```python
from build123d import *

# Parameters (mm, degrees)
F1_DEPTH = 2


# Not quite as in the source:
# - a feature names something its author has since deleted; it is built from what else it names


with BuildPart() as f1:
    # F0 (on Top) → F1 (new body)
    with BuildSketch(Plane.XY):
        Polygon((27.5, 51.9615242271), (-27.5, 51.9615242271), (-27.5, 47.6313972081), (-25.5, 46.4766966698), (-25.5, 49.9615242271), (25.5, 49.9615242271), (25.5, 46.4766966698), (27.5, 47.6313972081), align=None)
        Polygon((-25.5, 46.4766966698), (-27.5, 47.6313972081), (-27.5, 45.3219961314), (-25.5, 44.167295593), align=None)
        Polygon((-27.5, 45.3219961314), (-27.5, 47.6313972081), (-31.25, 49.7964607176), (-58.75, 2.1650635095), (-55, 0), (-53, 1.1547005384), (-56.0179491924, 2.897114317), (-30.5179491924, 47.06440991), align=None)
        Polygon((31.25, 49.7964607176), (27.5, 47.6313972081), (27.5, 45.3219961314), (30.5179491924, 47.06440991), (56.0179491924, 2.897114317), (53, 1.1547005384), (55, 0), (58.75, 2.1650635095), align=None)
        Polygon((27.5, 45.3219961314), (27.5, 47.6313972081), (25.5, 46.4766966698), (25.5, 44.167295593), align=None)
        Polygon((-25.5, 44.167295593), (-27.5, 45.3219961314), (-27.5, 15.8771324027), (-25.5, 17.0318329411), align=None)
        Polygon((25.5, 44.167295593), (25.5, 46.4766966698), (0, 31.7542648054), (2, 30.5995642671), align=None)
        Polygon((-25.5, 17.0318329411), (-27.5, 15.8771324027), (-27.5, 13.567731326), (-25.5, 14.7224318643), align=None)
        Polygon((2, 30.5995642671), (0, 31.7542648054), (-2, 30.5995642671), (0, 29.4448637287), align=None)
        Polygon((-25.5, 14.7224318643), (-27.5, 13.567731326), (-27.5, -13.567731326), (-25.5, -14.7224318643), align=None)
        Polygon((-2, 30.5995642671), (-25.5, 17.0318329411), (-25.5, 14.7224318643), (0, 29.4448637287), align=None)
        Polygon((-53, -1.1547005384), (-55, 0), (-58.75, -2.1650635095), (-31.25, -49.7964607176), (-27.5, -47.6313972081), (-27.5, -45.3219961314), (-30.5179491924, -47.06440991), (-56.0179491924, -2.897114317), align=None)
        Polygon((-53, 1.1547005384), (-55, 0), (-53, -1.1547005384), (-51, 0), align=None)
        Polygon((25.5, 17.0318329411), (2, 30.5995642671), (0, 29.4448637287), (25.5, 14.7224318643), align=None)
        Polygon((53, -1.1547005384), (55, 0), (53, 1.1547005384), (51, 0), align=None)
        Polygon((58.75, -2.1650635095), (55, 0), (53, -1.1547005384), (56.0179491924, -2.897114317), (30.5179491924, -47.06440991), (27.5, -45.3219961314), (27.5, -47.6313972081), (31.25, -49.7964607176), align=None)
        Polygon((-25.5, -14.7224318643), (-27.5, -13.567731326), (-27.5, -15.8771324027), (-25.5, -17.0318329411), align=None)
        Polygon((-27.5, -15.8771324027), (-27.5, -13.567731326), (-51, 0), (-53, -1.1547005384), align=None)
        Polygon((27.5, 15.8771324027), (25.5, 17.0318329411), (25.5, 14.7224318643), (27.5, 13.567731326), align=None)
        Polygon((51, 0), (53, 1.1547005384), (27.5, 15.8771324027), (27.5, 13.567731326), align=None)
        Polygon((0, -29.4448637287), (-25.5, -14.7224318643), (-25.5, -17.0318329411), (-2, -30.5995642671), align=None)
        Polygon((27.5, 13.567731326), (25.5, 14.7224318643), (25.5, -14.7224318643), (27.5, -13.567731326), align=None)
        Polygon((2, -30.5995642671), (0, -29.4448637287), (-2, -30.5995642671), (0, -31.7542648054), align=None)
        Polygon((25.5, -14.7224318643), (0, -29.4448637287), (2, -30.5995642671), (25.5, -17.0318329411), align=None)
        Polygon((-27.5, -45.3219961314), (-27.5, -47.6313972081), (-25.5, -46.4766966698), (-25.5, -44.167295593), align=None)
        Polygon((-25.5, -46.4766966698), (-27.5, -47.6313972081), (-27.5, -51.9615242271), (27.5, -51.9615242271), (27.5, -47.6313972081), (25.5, -46.4766966698), (25.5, -49.9615242271), (-25.5, -49.9615242271), align=None)
        Polygon((27.5, -13.567731326), (25.5, -14.7224318643), (25.5, -17.0318329411), (27.5, -15.8771324027), align=None)
        Polygon((25.5, -46.4766966698), (27.5, -47.6313972081), (27.5, -45.3219961314), (25.5, -44.167295593), align=None)
        Polygon((0, -31.7542648054), (-2, -30.5995642671), (-25.5, -44.167295593), (-25.5, -46.4766966698), align=None)
        Polygon((27.5, -15.8771324027), (25.5, -17.0318329411), (25.5, -44.167295593), (27.5, -45.3219961314), align=None)
    extrude(amount=F1_DEPTH)


solid = f1.part
```
The listing builds one solid part. Answer for the finished solid, in the listing's coordinates (mm). A direction names the side the tool comes from. Coordinates: 2 decimals unless noted, no trailing zeros. Write each loop counter-clockwise with the first axis right and the second up, starting at its lowest first coordinate (ties: lowest second). Pieces come first, ordered by that corner, then holes. Notation, with made-up numbers: (28, 35) - (62, 35) arc R26 ccw to (62, 49) - close; hole circle Ø2 at (37.25, 25). An arc over 180 degrees is marked (long way). Return JSON: item names as keys, results as strings. Group by question number.
1. A cutting plane is placed at C-C, the plane x = 45. Determine the outline of the cut face in (y, z).
2. A cutting plane is placed at B-B, the plane y = -11.5. Determine the outline of the cut face in (x, z).
3. A cutting plane is placed at D-D, the plane y = 36.5. Determine the outline of the cut face in (x, z).
4. A cutting plane is placed at A-A, the plane x = -6. Determine the outline of the cut face in (y, z).
5. Given pin 1 (1 mm diameter, centred on y = -50, z = 1, fed in from -X); pin 2 (0.6 mm diameter, centred on y = -20, z = 0.5, fed in from +X); pin 3 (0.6 mm diameter, centred on y = -49.5, z = 1.5, fed in from +X); pin 4 (12 mm diameter, centred on x = -11, y = -19.5, fed in from +Z), each flat-ended and moving along its own axis, determine where each tip first touches the part or whether it passes through.
6. Straight lines are drawn through the part: L1, parallel to X at y = 35, z = 1.75; L2, parallel to Y at x = -10.5, z = 1.4; L3, parallel to Y at x = 22.5, z = 0.15. For each, find the intervals that lie inside material, in ascending order.
7. Determine the mould class of faces 3 (the flat face through (-12.572, -22.187, 0.986)), 4 (the flat face through (45.19, 25.65, 0.99)), 5 (the flat face through (-45.19, -25.65, 0.99)) for opening direction X: released by +X, released by -X, zero draft, split by the parting line, or undercut.
8. Which of the six approach directions +Z, -Z, +X, -X, +Y, -Y give full straight-line access (tool end or side, diameter ignored) to faces 1 (the flat face through (-13, 23, 0)), 2 (the flat face through (-43.09, -25.29, 0.99))?
Ans:
{
 "1": {"outline": "(-25.98, 0) - (-21.98, 0) - (-21.98, 2) - (-25.98, 2) - close; (3.46, 0) - (5.77, 0) - (5.77, 2) - (3.46, 2) - close; (21.98, 0) - (25.98, 0) - (25.98, 2) - (21.98, 2) - close"},
 "2": {"outline": "(-53.36, 0) - (-51.05, 0) - (-51.05, 2) - (-53.36, 2) - close; (-35.08, 0) - (-31.08, 0) - (-31.08, 2) - (-35.08, 2) - close; (-27.5, 0) - (-25.5, 0) - (-25.5, 2) - (-27.5, 2) - close; (25.5, 0) - (27.5, 0) - (27.5, 2) - (25.5, 2) - close; (51.05, 0) - (53.36, 0) - (53.36, 2) - (51.05, 2) - close"},
 "3": {"outline": "(-38.93, 0) - (-36.62, 0) - (-36.62, 2) - (-38.93, 2) - close; (-27.5, 0) - (-25.5, 0) - (-25.5, 2) - (-27.5, 2) - close; (8.22, 0) - (12.22, 0) - (12.22, 2) - (8.22, 2) - close; (36.62, 0) - (38.93, 0) - (38.93, 2) - (36.62, 2) - close"},
 "4": {"outline": "(-51.96, 0) - (-49.96, 0) - (-49.96, 2) - (-51.96, 2) - close; (-35.22, 0) - (-32.91, 0) - (-32.91, 2) - (-35.22, 2) - close; (-28.29, 0) - (-25.98, 0) - (-25.98, 2) - (-28.29, 2) - close; (25.98, 0) - (28.29, 0) - (28.29, 2) - (25.98, 2) - close; (49.96, 0) - (51.96, 0) - (51.96, 2) - (49.96, 2) - close"},
 "5": {"pin 1": "x = -31.42", "pin 2": "x = 48.63", "pin 3": "x = 31.59", "pin 4": "z = 2"},
 "6": {"L1": "-39.79 to -37.48, -27.5 to -25.5, 5.62 to 9.62, 37.48 to 39.79", "L2": "-51.96 to -49.96, -37.82 to -35.51, -25.69 to -23.38, 23.38 to 25.69, 49.96 to 51.96", "L3": "-51.96 to -49.96, -18.76 to -16.45, 16.45 to 18.76, 42.44 to 44.74, 49.96 to 51.96"},
 "7": {"face 3": "undercut", "face 4": "released by +X", "face 5": "released by -X"},
 "8": {"face 1": "-Z, +X, -X, +Y, -Y", "face 2": "+Z, -Z"}
}
